Source: CAD feature listing. Evaluate the final solid. Frame: model axes, mm. A direction names the side the tool comes from. Give positions to 0.01 mm unless a question says otherwise; leave off trailing zeros. Write each loop counter-clockwise with the first axis right and the second up, starting at its lowest first coordinate (ties: lowest second). Pieces come first, ordered by that corner, then holes. Notation, with made-up numbers: (75.25, 2) - (105.25, 2) arc R38 ccw to (105.25, 40) - close; hole circle Ø6 at (-7.75, 14.5). An arc over 180 degrees is marked (long way). One line per question, with ' | ' between items. Start each with the question number.
(1) Pin query (flat end, axial travel): pin 1 (4 mm diameter, centred on x = 8, z = 1.5, fed in from +Y); pin 2 (1.5 mm diameter, centred on x = 14, z = 10.5, fed in from +Y). Return the tip coordinate at first contact, or that it passes through.
(2) Section C-C, the plane y = 2.75. State how many separate pieces and enclosed holes the cut face has, plus the area to 3 significant figures.
(3) Access query for faces 5 (the cylindrical face through (15.43, 0.9, -0.63)), 6 (the flat face through (8, 1.5, -1)), 7 (the flat face through (8, 0, -15)). Directions: +Z, -Z, +X, -X, +Y, -Y. A direction counts if a zero-diameter tool reaches every point of the face in a straight line with its end or side. Return the directions, or none.
(4) Section B-B, the plane z = 0.75. Return loops of the section in (x, y).
(5) Draft query along Z for faces 1 (the cylindrical face through (8.23, 1.47, 7.66)), 2 (the flat face through (8, 2, 5.202)), 3 (the cylindrical face through (0.374, 3.546, -11.773)), 4 (the cylindrical face through (8.11, 1.31, 14.71)). Return one class per face: +Z half, -Z half, draft (parallel to the pull), parting line (faces both ways), or undercut.
(6) Section A-A, the plane x = 6. Return loops of the section in (y, z), plus the area to 3 significant figures.
(7) Ray query, line 1 (Y direction, x = 13.75, z = -1.75); line 2 (Z direction, x = 3.5, y = 3.5); line 3 (Y direction, x = 7.5, z = -5). Return the intervals inside material, ascending. Write a range as [from, to].
```python
from build123d import *

# Parameters (mm, degrees)
F1_DEPTH = 16
F2_R     = 1.05
F3_DEPTH = 7.7105812745
F4_R     = 2


with BuildPart() as f1:
    # F0 (on Right) → F1 (new body)
    with BuildSketch(Plane.YZ):
        Polygon((-1.5, -15), (1.5, -15), (1.5, -7), (1.5, -3), (1.5, 5.2020410289), (1.5, 15), (-1.5, 15), align=None)
        Polygon((6.5, 5.2020410289), (1.5, 15), (1.5, 5.2020410289), align=None)
        Polygon((1.5, -7), (1.5, -15), (6.6618086312, -9.8381913688), (6.6618086312, -4.7058628306), (5.187990124, -5.3608932782), align=None)
    extrude(amount=F1_DEPTH)

    # F2 (on face) → F3 (cut, up to face)
    with BuildSketch(Plane(origin=(0, 7.2631977094, 3.7064850602), x_dir=(-1, 0, 0), z_dir=(0, 0.8907235428, 0.4545454545))):
        with Locations((-8, 7.1790349606)):
            Circle(F2_R)
    extrude(amount=-F3_DEPTH, mode=Mode.SUBTRACT)

    # F4
    f4_edges = [f1.edges().sort_by_distance(p)[0] for p in [
        (16, 1.5, -0.898979),
        (0, 1.5, -0.898979),
        (16, 4, 10.101021),
        (0, 4, 10.101021),
        (8, 6.5, 5.202041),
        (8, 6.661809, -9.838191),
        (16, 4.080904, -12.419096),
        (0, 4.080904, -12.419096),
        (16, 4.080904, -5.852931),
        (0, 4.080904, -5.852931),
        (8, 1.5, 15),
        (8, 1.5, -15),
    ]]
    fillet(f4_edges, radius=F4_R)


solid = f1.part
```
Check sheet entries:
1) pin 1: y = 1.5 | pin 2: y = 4.18
2) separate pieces: 2 | enclosed holes: 1 | area: 222 mm²
3) face 5: +X | face 6: +X, -X | face 7: -Z, +X, -X, +Y, -Y
4) outline: (0, -1.5) - (16, -1.5) - (16, -0.5) arc R2 ccw to (14, 1.5) - (2, 1.5) arc R2 ccw to (0, -0.5) - close
5) face 1: undercut | face 2: undercut | face 3: -Z half | face 4: +Z half
6) outline: (-1.5, -15) - (0.67, -15) arc R2 ccw to (2.09, -14.41) - (6.08, -10.42) arc R2 ccw to (6.66, -9.01) - (6.66, -4.71) - (1.5, -7) - (1.5, 5.2) - (3.23, 5.2) arc R2 ccw to (5.02, 8.11) - (2.06, 13.91) arc R2 ccw to (0.28, 15) - (-1.5, 15) - close | area: 146 mm²
7) line 1: [-1.5, 1.5] | line 2: [-13, -6.11], [5.22, 11.08] | line 3: [-1.5, 1.5], [6, 6.66]
